```python
from build123d import *

# Parameters (mm, degrees)
F0_W     = 159.953385
F0_H     = 135.459002
F1_DEPTH = 25.4
F2_W     = 23.394922
F2_H     = 22.785936
F3_DEPTH = 101.6
F4_W     = 29.928277
F4_H     = 18.628203
F5_DEPTH = 50.8
F6_W     = 136.795349
F6_H     = 112.584971
F7_DEPTH = 50.8
F8_W     = 29.928277
F8_H     = 18.628203
F9_DEPTH = 50.8


with BuildPart() as f1:
    # F0 (on Front) → F1 (new body)
    with BuildSketch(Plane.XZ):
        with Locations((-0.262774, 11.529313)):
            Rectangle(F0_W, F0_H)
    extrude(amount=F1_DEPTH)

    # F2 (on Top) → F3 (join)
    with BuildSketch(Plane.XY):
        with Locations((2.348405, -11.392968)):
            Rectangle(F2_W, F2_H)
    extrude(amount=F3_DEPTH)

    # F4 (on Right) → F5 (join)
    with BuildSketch(Plane.YZ):
        with Locations((-10.842666, 105.735038)):
            Rectangle(F4_W, F4_H)
    extrude(amount=F5_DEPTH)

    # F6 (on Front) → F7 (join)
    with BuildSketch(Plane.XZ):
        with Locations((0.471081, 11.709642)):
            Rectangle(F6_W, F6_H)
    extrude(amount=F7_DEPTH)

    # F8 (on face) → F9 (join)
    with BuildSketch(Plane(origin=(0, 0, 0), x_dir=(0, -1, 0), z_dir=(-1, 0, 0))):
        with Locations((10.842666, 105.735038)):
            Rectangle(F8_W, F8_H)
    extrude(amount=F9_DEPTH)


solid = f1.part
```
Work out the finished part from the listing and answer in its coordinate system (mm). A direction names the side the tool comes from. Round coordinates to 2 decimals unless told otherwise and drop trailing zeros. Loops run counter-clockwise (first coordinate to the right, second up) from the corner with the lowest first, then second, coordinate; pieces in that order, holes last. Notation, with made-up numbers: (88.25, -17.75) -> (105.25, -17.75) arc R23 cw to (105.25, -8.75) -> close; hole circle Ø5 at (-6, -15). An arc over 180 degrees is marked (long way). Write each question's results on one line, items separated by ' | '. Start each with the question number.
1. Section D-D (y = -12.5) is taken. Determine the outline of the cut face in (x, z), plus the area to 3 significant figures.
2. A tool of negligible diameter and unlimited length cuts with its end or side. For faces 4 (the face through (68.869, -38, 11)), 5 (the face through (-50.8, -11, 106)), 6 (the face through (2, -22.786, 88)), 7 (the face through (0, -38, -44.583)), from which of +Z, -Z, +X, -X, +Y, -Y can it reach the whole face along a straight path? Write none if from no direction.
3. Section A-A (x = -35.5) is taken. Determine the outline of the cut face in (y, z), plus the area to 3 significant figures.
4. Section C-C (x = 1.5) is taken. Determine the outline of the cut face in (y, z), plus the area to 3 significant figures.
5. Given pin 1 Ø3 at (y, z) = (-45, 18.5) entering from -X; pin 2 Ø19 at (y, z) = (-9, 90) entering from +X; pin 3 Ø13.5 at (x, z) = (0, 88.5) entering from -Y, each flat-ended and moving along its own axis, determine where each tip first touches the part or whether it passes through.
6. Section B-B (z = 35) is taken. Determine the outline of the cut face in (x, y), plus the area to 3 significant figures.
7. For a pull along Z with two mould halves and no side action, classify faces 1 (the face through (1, -11, 115.049)), 2 (the face through (-1, -24, 79.259)), 3 (the face through (0, -50.8, 12)) as +Z half, -Z half, draft (parallel to the pull), parting line (faces both ways), or undercut.
8. Find the intervals of material crossed by probe 1 along Z at (x, y) = (-32, -17); probe 2 along Y at (x, z) = (-10, -40); probe 3 along X at (y, z) = (-35, -39.5), in increasing order. Write a range as from..to.
Evaluation:
1) outline: (-80.24, -56.2) -> (79.71, -56.2) -> (79.71, 79.26) -> (14.05, 79.26) -> (14.05, 96.42) -> (50.8, 96.42) -> (50.8, 115.05) -> (-50.8, 115.05) -> (-50.8, 96.42) -> (-9.35, 96.42) -> (-9.35, 79.26) -> (-80.24, 79.26) -> close | area: 24,000 mm2
2) face 4: +Z, -Z, +X, -Y | face 5: +Z, -X, +Y, -Y | face 6: +X, -X, -Y | face 7: -Z, +X, -X, -Y
3) outline: (-50.8, -44.58) -> (-25.4, -44.58) -> (-25.4, -56.2) -> (0, -56.2) -> (0, 79.26) -> (-25.4, 79.26) -> (-25.4, 68) -> (-50.8, 68) -> close; (-25.81, 96.42) -> (4.12, 96.42) -> (4.12, 115.05) -> (-25.81, 115.05) -> close | area: 6,860 mm2
4) outline: (-50.8, -44.58) -> (-25.4, -44.58) -> (-25.4, -56.2) -> (0, -56.2) -> (0, 96.42) -> (4.12, 96.42) -> (4.12, 115.05) -> (-25.81, 115.05) -> (-25.81, 96.42) -> (-22.79, 96.42) -> (-22.79, 79.26) -> (-25.4, 79.26) -> (-25.4, 68) -> (-50.8, 68) -> close | area: 7,250 mm2
5) pin 1: stops at x = -67.93 | pin 2: stops at x = 50.8 | pin 3: stops at y = -22.79
6) outline: (-80.24, -25.4) -> (-67.93, -25.4) -> (-67.93, -50.8) -> (68.87, -50.8) -> (68.87, -25.4) -> (79.71, -25.4) -> (79.71, 0) -> (-80.24, 0) -> close | area: 7,540 mm2
7) face 1: +Z half | face 2: undercut | face 3: draft
8) probe 1: z = -56.2..79.26, 96.42..115.05 | probe 2: y = -50.8..0 | probe 3: x = -67.93..68.87
